For this review, take the finished solid that the model builds, in its own axes (mm). Face numbers are marked on the shaded views. A direction names the side the tool comes from. Give positions to 0.01 mm unless a question says otherwise; leave off trailing zeros. Loops run counter-clockwise (first coordinate to the right, second up) from the corner with the lowest first, then second, coordinate; pieces in that order, holes last. Notation, with made-up numbers: M -18.75,33 L 4.25,33 A15 cw 4.25,40 Z; hole C 31,67.25 d1. An arc over 180 degrees is marked long. Use CSV: the item, a comma, the result in double quotes. Start each with the question number.
1. Tool access review of the marked faces 4, 5, 6 and 7: name each direction out of +Z, -Z, +X, -X, +Y, -Y from which nothing blocks a thin tool from reaching the whole face with its end or side.
2. The part is to be moulded in two halves that separate along X. For the marked faces 1, 2 and 3, say which applies: pulls with the +X half, pulls with the -X half, needs draft (parallel to the pull), parting line crosses it, or undercut.
3. Take a section at D-D, the plane x = -53.5. Write out the cut boundary in (y, z).
4. Take a section at A-A, the plane z = 15.25. Write out the cut boundary in (x, y).
5. Take a section at B-B, the plane x = -35.43. Write out the cut boundary in (y, z).
6. To check wall thickness, follow line 1 (Y direction, x = -30.68, z = 20.5); line 2 (Y direction, x = -33, z = 19.5); line 3 (X direction, y = 20.5, z = 15.5). State the ranges of each line that lie inside material, in increasing order. Write a range as [from, to].
7. Insertion check: P1, Ø3, axis at x = -58, z = 14, coming from the +Y side; P2, Ø3, axis at y = -2.5, z = 15, coming from the -X side; P3, Ø1.1, axis at x = -59, z = 17.5, coming from the -Y side; P4, Ø1.5, axis at x = -40.18, y = 16.18, coming from the -Z side. Each pin has a flat end and moves straight along its axis. Give the tip position at first contact, or say it passes through.
8. Take a section at C-C, the plane y = 23.5. Write out the cut boundary in (x, z), and give its area (3 significant figures).
Autodesk Inventor part; units mm, degrees
ref_plane "Work Plane1" through (-56.3599, 0, 22) normal (0, 0, -1) x (-1, 0, 0)
ref_plane "YZ Plane" through (0, 0, 0) normal (1, 0, 0) x (0, 1, 0)
ref_plane "XZ Plane" through (0, 0, 0) normal (0, 1, 0) x (-1, 0, 0)
ref_plane "Work Plane1" through (-56.3599, 0, 22) normal (0, 0, -1) x (-1, 0, 0)
sketch "Sketch1" plane through (-56.3599, 0, 22) normal (0, 0, -1) x (-1, 0, 0)
  line L0 (-4.0299, -0.3538) -> (-2.2322, 1.4439) construction
  arc A0 (-1.4439, 2.2322) -> (-2.2322, 1.4439) centre (-0.9299, 0.9299) ccw construction
  line L1 (-1.4439, 2.2322) -> (0.3538, 4.0299) construction
  line L2 (-37.8299, 42.8299) -> (-37.8299, 37.8299) construction
  line L3 (-37.8299, 37.8299) -> (-42.9208, 37.8299) construction
  line L4 (-37.8299, 42.2137) -> (-37.8299, 45.8299) construction
  line L5 (-37.8299, 45.8299) -> (-4.0299, 45.8299) construction
  line L6 (-4.0299, 45.8299) -> (-4.0299, 42.2137) construction
  line L7 (-4.0299, 4.0299) -> (0.3538, 4.0299)
  circle A1 centre (-20.9299, 20.9299) radius 17.5
  line L8 (-20.9299, 58.9723) -> (17.1124, 20.9299) construction
  line L9 (17.1124, 20.9299) -> (-20.9299, -17.1124) construction
  line L10 (-20.9299, -17.1124) -> (-58.9723, 20.9299) construction
  line L11 (-58.9723, 20.9299) -> (-20.9299, 58.9723) construction
  line L12 (-20.9299, 58.9723) -> (-20.9299, -17.1124) construction
  line L13 (17.1124, 20.9299) -> (-58.9723, 20.9299) construction
  line L14 (-20.9299, 58.9723) -> (32.8701, 58.9723) construction
  line L15 (-43.4299, 43.4299) -> (1.5701, 43.4299) construction
  line L16 (1.5701, 43.4299) -> (1.5701, -1.5701) construction
  line L17 (1.5701, -1.5701) -> (-43.4299, -1.5701) construction
  line L18 (-43.4299, -1.5701) -> (-43.4299, 43.4299) construction
  line L19 (-43.4299, 43.4299) -> (1.5701, -1.5701) construction
  line L20 (1.5701, 43.4299) -> (-43.4299, -1.5701) construction
  line L21 (-43.4299, 5.3876) -> (-43.4299, 36.4723)
  line L22 (-43.4299, 36.4723) -> (-36.4723, 43.4299)
  line L23 (-36.4723, 43.4299) -> (-5.3876, 43.4299)
  line L24 (-5.3876, 43.4299) -> (1.5701, 36.4723)
  line L25 (1.5701, 36.4723) -> (1.5701, 5.3876)
  line L26 (1.5701, 5.3876) -> (-5.3876, -1.5701)
  line L27 (-5.3876, -1.5701) -> (-36.4723, -1.5701)
  line L28 (-36.4723, -1.5701) -> (-43.4299, 5.3876)
  line L29 (-4.0299, 42.2137) -> (-37.8299, 42.2137)
  line L30 (-4.0299, -0.3538) -> (-4.0299, 4.0299)
  circle A2 centre (-20.9299, 20.9299) radius 1.5
  line L31 (-10.9299, 10.9299) -> (-30.9299, 10.9299) construction
  line L32 (-30.9299, 10.9299) -> (-30.9299, 30.9299) construction
  line L33 (-30.9299, 30.9299) -> (-10.9299, 30.9299) construction
  line L34 (-10.9299, 30.9299) -> (-10.9299, 10.9299) construction
  line L35 (-10.9299, 10.9299) -> (-30.9299, 30.9299) construction
  line L36 (-30.9299, 10.9299) -> (-10.9299, 30.9299) construction
  circle A3 centre (-30.9299, 30.9299) radius 1.4
  circle A4 centre (-30.9299, 10.9299) radius 1.4
  circle A5 centre (-10.9299, 10.9299) radius 1.4
  line L37 (-45.8299, 37.8299) -> (-42.0723, 37.8299) construction
  line L38 (-42.1723, 37.7299) -> (-45.8299, 37.7299)
  line L39 (-45.8299, 37.7299) -> (-45.8299, 4.1299)
  line L40 (-45.8299, 4.1299) -> (-42.1723, 4.1299)
  line L41 (-42.1723, 4.1299) -> (-42.1723, 37.7299)
  line L42 (-45.8299, 4.0299) -> (-42.0723, 4.0299) construction
  line L43 (-45.8299, 37.8299) -> (-42.0723, 37.8299)
  line L44 (-37.7299, 45.8299) -> (-4.1299, 45.8299)
  line L45 (-4.1299, 45.8299) -> (-4.1299, 42.1723)
  line L46 (-4.1299, 42.1723) -> (-37.7299, 42.1723)
  line L47 (-37.7299, 42.1723) -> (-37.7299, 45.8299)
  line L48 (0.4701, 37.8299) -> (0.4701, 4.0299) construction
  line L49 (0.4701, 4.0299) -> (3.9701, 4.0299) construction
  line L50 (3.9701, 37.8299) -> (3.9701, 4.0299) construction
  line L51 (0.4701, 37.8299) -> (3.9701, 37.8299) construction
  line L52 (-45.8299, -3.9701) -> (-4.0299, -3.9701) construction
  line L53 (0.3124, 37.7299) -> (3.9701, 37.7299)
  line L54 (3.9701, 37.7299) -> (3.9701, 4.1299)
  line L55 (3.9701, 4.1299) -> (0.3124, 4.1299)
  line L56 (0.3124, 4.1299) -> (0.3124, 37.7299)
  line L57 (-4.1713, -0.3538) -> (-37.7299, -0.3538)
  line L58 (-37.7299, -0.3538) -> (-37.7299, -3.9701)
  line L59 (-37.7299, -3.9701) -> (-4.1713, -3.9701)
  line L60 (-4.1713, -3.9701) -> (-4.1713, -0.3538)
  point P0 (-37.8299, 4.0299)
  dimension "d18" = 53.8
  dimension "d19" = 45
  dimension "d20" = 53.8
  dimension "d21" = 45
  dimension "d22" = 45
  dimension "d30" = 20
  dimension "d31" = 20
  dimension "d32" = 2.8
  dimension "d33" = 2.8
  dimension "d34" = 2.8
  dimension "d35" = 3
  dimension "d36" = 0.1
  dimension "d37" = 0.1
  dimension "d38" = 0.1
  dimension "d39" = 0.1
extrude "Extrusion1" add sketch "Sketch1" along normal blind 12 contours L30 L26 L57 L28 L41 L22 L46 L24 L56 L7 | L7 L26 L30 | L56 L24 L25 L26 | L26 L25 L24 L53 L54 L55 | L60 L59 L58 L57 L28 L27 L26 | L26 L27 L28 L57 | L46 L22 L29 L24 | L24 L29 L45 | L40 L39 L38 L22 L21 L28 | L28 L21 L22 L41 | L29 L22 L23 L24 | L24 L23 L22 L29 L47 L44 L45 | L47 L29 L22 | A1 | A2 | A3 | A4 | A5
sketch "Skizze4" plane through (-56.3599, 0, 10) normal (0, 0, -1) x (-1, 0, 0)
  line L0 (-37.7299, 42.1723) -> (-42.1723, 37.7299)
  line L1 (-42.1723, 37.7299) -> (-45.8299, 37.7299)
  line L2 (-45.8299, 37.7299) -> (-45.8299, 4.1299) construction
  line L3 (-45.8299, 4.1299) -> (-42.1723, 4.1299)
  line L4 (-42.1723, 4.1299) -> (-37.6885, -0.3538)
  line L5 (-37.6885, -0.3538) -> (-37.7299, -0.3538)
  line L6 (-37.7299, -0.3538) -> (-37.7299, -3.9701)
  line L7 (-37.7299, -3.9701) -> (-4.1713, -3.9701) construction
  line L8 (-4.1713, -3.9701) -> (-4.1713, -0.3538)
  line L9 (-4.1713, -0.3538) -> (0.3124, 4.1299)
  line L10 (0.3124, 4.1299) -> (3.9701, 4.1299)
  line L11 (3.9701, 4.1299) -> (3.9701, 37.7299) construction
  line L12 (3.9701, 37.7299) -> (0.3124, 37.7299)
  line L13 (0.3124, 37.7299) -> (-4.1299, 42.1723)
  line L14 (-4.1299, 42.1723) -> (-4.1299, 45.8299)
  line L15 (-4.1299, 45.8299) -> (-37.7299, 45.8299) construction
  line L16 (-37.7299, 45.8299) -> (-37.7299, 42.1723)
  line L17 (-37.9299, 46.0299) -> (-3.9299, 46.0299) construction
  line L18 (-3.9299, 46.0299) -> (-3.9299, 42.2551)
  line L19 (-3.9299, 42.2551) -> (0.3953, 37.9299)
  line L20 (0.3953, 37.9299) -> (4.1701, 37.9299)
  line L21 (4.1701, 37.9299) -> (4.1701, 3.9299) construction
  line L22 (4.1701, 3.9299) -> (0.3953, 3.9299)
  line L23 (0.3953, 3.9299) -> (-3.9713, -0.4367)
  line L24 (-3.9713, -0.4367) -> (-3.9713, -4.1701)
  line L25 (-3.9713, -4.1701) -> (-37.9299, -4.1701) construction
  line L26 (-37.9299, -4.1701) -> (-37.9299, -0.3953)
  line L27 (-37.9299, -0.3953) -> (-42.2551, 3.9299)
  line L28 (-42.2551, 3.9299) -> (-46.0299, 3.9299)
  line L29 (-46.0299, 3.9299) -> (-46.0299, 37.9299) construction
  line L30 (-46.0299, 37.9299) -> (-42.2551, 37.9299)
  line L31 (-42.2551, 37.9299) -> (-37.9299, 42.2551)
  line L32 (-37.9299, 42.2551) -> (-37.9299, 46.0299)
  line L33 (-45.8299, 37.7299) -> (-45.8299, 37.9299)
  line L34 (-4.1299, 45.8299) -> (-37.7299, 45.8299)
  line L35 (-37.7299, 45.8299) -> (-37.9299, 45.8299)
  line L36 (-4.1299, 45.8299) -> (-3.9299, 45.8299)
  line L37 (3.9701, 37.7299) -> (3.9701, 37.9299)
  line L38 (3.9701, 4.1299) -> (3.9701, 37.7299)
  line L39 (3.9701, 4.1299) -> (3.9701, 3.9299)
  line L40 (-4.1713, -3.9701) -> (-3.9713, -3.9701)
  line L41 (-37.7299, -3.9701) -> (-37.9299, -3.9701)
  line L42 (-45.8299, 4.1299) -> (-45.8299, 3.9299)
  point P0 (-56.3599, 0)
  dimension "d40" = 0.2
extrude "IM_offset" add sketch "Skizze4" against normal up to surface (12 mm away)
ref_plane "Arbeitsebene5" through (-35.4299, 3.9299, 22) normal (-1, 0, 0) x (0, 0, 1)
ref_plane "Arbeitsebene6" through (-18.4299, 20.9299, 22) normal (0, 1, 0) x (-1, 0, 0)
sketch "Skizze31" plane through (-56.3599, 0, 10) normal (0, 0, -1) x (-1, 0, 0)
  line L0 (3.9701, 3.9299) -> (3.9701, 37.9299)
  line L1 (3.9701, 37.9299) -> (0.3953, 37.9299)
  line L2 (0.3953, 37.9299) -> (-3.9299, 42.2551)
  line L3 (-3.9299, 42.2551) -> (-3.9299, 45.8299)
  line L4 (-3.9299, 45.8299) -> (-37.9299, 45.8299)
  line L5 (-37.9299, 45.8299) -> (-37.9299, 42.2551)
  line L6 (-37.9299, 42.2551) -> (-42.2551, 37.9299)
  line L7 (-42.2551, 37.9299) -> (-45.8299, 37.9299)
  line L8 (-45.8299, 37.9299) -> (-45.8299, 3.9299)
  line L9 (-42.2551, 3.9299) -> (-45.8299, 3.9299)
  line L10 (-37.9299, -0.3953) -> (-42.2551, 3.9299)
  line L11 (-37.9299, -3.9701) -> (-37.9299, -0.3953)
  line L12 (-3.9713, -3.9701) -> (-37.9299, -3.9701)
  line L13 (-3.9713, -3.9701) -> (-3.9713, -0.4367)
  line L14 (-3.9713, -0.4367) -> (0.3953, 3.9299)
  line L15 (0.3953, 3.9299) -> (3.9701, 3.9299)
  line L16 (-11.9299, 27.4299) -> (-27.4299, 27.4299)
  line L17 (-11.9299, 14.4299) -> (-11.9299, 27.4299)
  line L18 (-27.4299, 14.4299) -> (-11.9299, 14.4299)
  line L19 (-27.4299, 27.4299) -> (-27.4299, 14.4299)
  circle A0 centre (-20.9299, 20.9299) radius 4.5
  circle A1 centre (-25.6799, 25.6799) radius 0.75
  circle A2 centre (-25.6799, 16.1799) radius 0.75
  circle A3 centre (-16.1799, 16.1799) radius 0.75
  circle A4 centre (-16.1799, 25.6799) radius 0.75
  line L20 (-27.6299, 14.2299) -> (-11.7299, 14.2299)
  line L21 (-11.7299, 14.2299) -> (-11.7299, 27.6299)
  line L22 (-11.7299, 27.6299) -> (-27.6299, 27.6299)
  line L23 (-27.6299, 27.6299) -> (-27.6299, 14.2299)
  point P0 (-56.3599, 0)
  dimension "d184" = 0.2
extrude "Extrusion26" cut sketch "Skizze31" against normal blind 10 contours L17 L18 L19 L16 | A0 | A1 | A2 | A3 | A4 | L23 L22 L21 L20
sketch "Skizze32" plane through (-56.3599, 0, 22) normal (0, 0, 1) x (1, 0, 0)
  circle A0 centre (20.9299, 20.9299) radius 4.5
  circle A1 centre (25.6799, 25.6799) radius 1.25
  circle A2 centre (16.1799, 16.1799) radius 1.25
  circle A3 centre (25.6799, 16.1799) radius 1.25
  circle A4 centre (16.1799, 25.6799) radius 1.25
  line L0 (14.4299, 27.4299) -> (27.4299, 27.4299)
  line L1 (27.4299, 27.4299) -> (27.4299, 14.4299)
  line L2 (27.4299, 14.4299) -> (14.4299, 14.4299)
  line L3 (14.4299, 14.4299) -> (14.4299, 27.4299)
  point P0 (56.3599, 0)
extrude "Extrusion27" cut sketch "Skizze32" against normal blind 10 contours A0 | A1 | A2 | A3 | A4
properties part number "20_Cube_Insert_Lasertack_mount_v3"
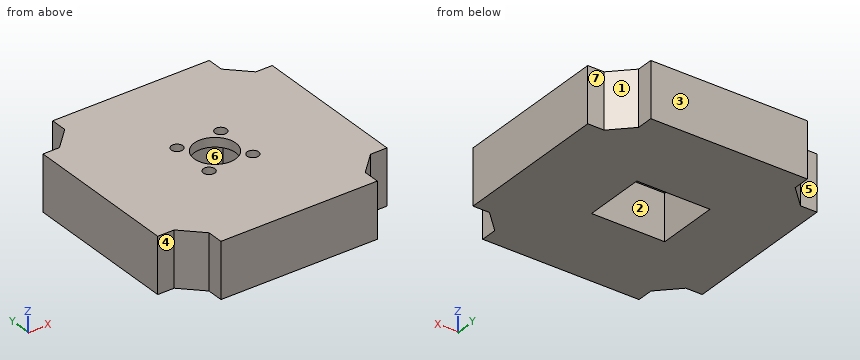
Result set:
1,face 4,"+Z, -Z, -X, -Y"
1,face 5,"+Z, -Z, -X, +Y"
1,face 6,"-Z"
1,face 7,"+Z, -Z, +X, +Y"
2,face 1,"pulls with the +X half"
2,face 2,"undercut"
2,face 3,"needs draft"
3,outline,"M 0.67,10 L 41.19,10 L 41.19,22 L 0.67,22 Z"
4,outline,"M -60.33,3.93 L -56.76,3.93 L -52.39,-0.44 L -52.39,-3.97 L -18.43,-3.97 L -18.43,-0.4 L -14.1,3.93 L -10.53,3.93 L -10.53,37.93 L -14.1,37.93 L -18.43,42.26 L -18.43,45.83 L -52.43,45.83 L -52.43,42.26 L -56.76,37.93 L -60.33,37.93 Z; hole M -44.63,14.23 L -28.73,14.23 L -28.73,27.63 L -44.63,27.63 Z"
5,outline,"M -3.97,10 L 14.23,10 L 14.23,20 L 16.43,20 L 16.43,22 L -3.97,22 Z; M 25.43,20 L 27.63,20 L 27.63,10 L 45.83,10 L 45.83,22 L 25.43,22 Z"
6,line 1,"[-3.97, 14.93], [17.43, 24.43], [26.93, 45.83]"
6,line 2,"[-3.97, 14.23], [27.63, 45.83]"
6,line 3,"[-60.33, -44.63], [-28.73, -10.53]"
7,P1,"y = 38.19"
7,P2,"x = -52.39"
7,P3,"y = 3.93"
7,P4,"through"
8,outline,"M -60.33,10 L -44.63,10 L -44.63,20 L -39.12,20 L -39.12,22 L -60.33,22 Z; M -31.74,20 L -28.73,20 L -28.73,10 L -10.53,10 L -10.53,22 L -31.74,22 Z"
8,area,"424 mm2"
